For this review, take the finished solid that the model builds, in its own axes (mm). Face numbers are marked on the shaded views. Give positions to 0.01 mm unless a question says otherwise; leave off trailing zeros. Order: outer loops, then holes, each group sorted by start corner. A loop starts at its lowest first (then second) coordinate and runs counter-clockwise, first axis right, second up. Notation, with made-up numbers: M 28,-2 L 73,-2 A28 ccw 73,25 Z; hole C 65.25,44.5 d2. An arc over 180 degrees is marked long. Answer as CSV lines item,"result". Start each with the question number.
1. We need section D-D, the plane y = -12. Give the boundary of the cut face in (x, z).
2. We need section A-A, the plane z = 1.5. Give the boundary of the cut face in (x, y), and give its area (3 significant figures).
3. Mouldability with a two-part tool opening along X and no side actions: class the marked faces 1 and 2 as pulls with the +X half, pulls with the -X half, needs draft (parallel to the pull), parting line crosses it, or undercut.
4. We need section B-B, the plane y = 15. Give the boundary of the cut face in (x, z), and give its area (3 significant figures).
5. For line 1 along Y through (x, z) = (-36, 7); line 2 along X through (y, z) = (43, 6); line 3 along X through (y, z) = (22.5, 1.25), list the stretches that pass through material, from the lowest coordinate up.
6. We need section C-C, the plane x = -28. Give the boundary of the cut face in (y, z).
7. Clearance check with a flat-ended pin moving along its axis: P1, Ø4, axis at x = -10, y = -17, coming from the +Z side. State where the tip first meets the part, or that it passes through.
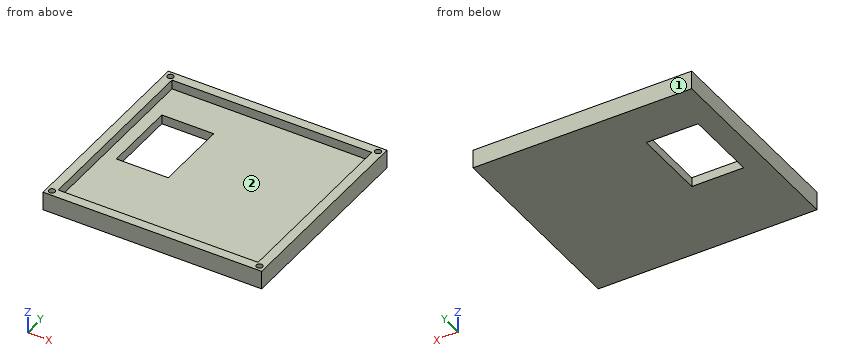
Autodesk Fusion 360 part; units mm, degrees
sketch "Sketch1" plane through (0, 0, 0) normal (0, 0, 1) x (1, 0, 0)
  line L0 (53.7502, -49.9897) -> (-53.7502, -49.9897)
  line L1 (-53.7502, -49.9897) -> (-53.7502, 49.9897)
  line L2 (-53.7502, 49.9897) -> (53.7502, 49.9897)
  line L3 (53.7502, 49.9897) -> (53.7502, -49.9897)
  line L4 (53.7502, -49.9897) -> (-53.7502, 49.9897) construction
  line L5 (-53.7502, -49.9897) -> (53.7502, 49.9897) construction
  line L6 (58.826, -55.0656) -> (-58.826, -55.0656)
  line L7 (-58.826, -55.0656) -> (-58.826, 55.0656)
  line L8 (-58.826, 55.0656) -> (58.826, 55.0656)
  line L9 (58.826, 55.0656) -> (58.826, -55.0656)
  circle A0 centre (-55.826, 52.0656) radius 1.7
  circle A1 centre (-55.826, 52.0656) radius 1.7
  circle A2 centre (55.826, 52.0656) radius 1.7
  circle A3 centre (55.826, -52.0656) radius 1.7
  circle A4 centre (-55.826, -52.0656) radius 1.7
  line L10 (-47.1513, 30.2997) -> (-19.2113, 30.2997)
  line L11 (-19.2113, 30.2997) -> (-19.2113, -9.7053)
  line L12 (-19.2113, -9.7053) -> (-47.1513, -9.7053)
  line L13 (-47.1513, -9.7053) -> (-47.1513, 30.2997)
  dimension "d1" = 107.5004
  dimension "d2" = 99.9795
  dimension "d3" = -5.0758
  dimension "d4" = 3.4
  dimension "d5" = 3
  dimension "d6" = 3
  dimension "d7" = 3.4
  dimension "d8" = 3.4
  dimension "d9" = 3
  dimension "d10" = 3
  dimension "d11" = 3.4
  dimension "d12" = 3
  dimension "d13" = 3
  dimension "d14" = 3.4
  dimension "d15" = 3
  dimension "d16" = 3
  dimension "d17" = 6.5989
  dimension "d18" = 19.6901
  dimension "d19" = 27.94
  dimension "d20" = 40.005
extrude "Extrude1" add sketch "Sketch1" along normal blind 5 contours L0 L1 L2 L3
extrude "Extrude2" add sketch "Sketch1" along normal blind 10 contours L6 L7 L8 L9
extrude "Extrude3" add sketch "Sketch1" along normal blind 5 contours A0 A1 | A2 | A3 | A4
Result set:
1,outline,"M -58.83,0 L 58.83,0 L 58.83,10 L 53.75,10 L 53.75,5 L -53.75,5 L -53.75,10 L -58.83,10 Z"
2,outline,"M -58.83,-55.07 L 58.83,-55.07 L 58.83,55.07 L -58.83,55.07 Z; hole M -47.15,-9.71 L -19.21,-9.71 L -19.21,30.3 L -47.15,30.3 Z"
2,area,"11,800 mm2"
3,face 1,"needs draft"
3,face 2,"undercut"
4,outline,"M -58.83,0 L -47.15,0 L -47.15,5 L -53.75,5 L -53.75,10 L -58.83,10 Z; M -19.21,0 L 58.83,0 L 58.83,10 L 53.75,10 L 53.75,5 L -19.21,5 Z"
4,area,"499 mm2"
5,line 1,"-55.07 to -49.99, 49.99 to 55.07"
5,line 2,"-58.83 to -53.75, 53.75 to 58.83"
5,line 3,"-58.83 to -47.15, -19.21 to 58.83"
6,outline,"M -55.07,0 L -9.71,0 L -9.71,5 L -49.99,5 L -49.99,10 L -55.07,10 Z; M 30.3,0 L 55.07,0 L 55.07,10 L 49.99,10 L 49.99,5 L 30.3,5 Z"
7,P1,"z = 5"
